Design review of the part built by this model. Coordinates are the model's own, in mm. A direction names the side the tool comes from. Coordinates: 2 decimals unless noted, no trailing zeros. Write each loop counter-clockwise with the first axis right and the second up, starting at its lowest first coordinate (ties: lowest second). Pieces come first, ordered by that corner, then holes. Notation, with made-up numbers: (11, 84.25) - (17, 84.25) arc R24 ccw to (17, 114.25) - close; hole circle Ø2 at (43.5, 42). An arc over 180 degrees is marked (long way). Use a Markdown table: item, result.
from build123d import *

# Parameters (mm, degrees)
BASE_FLANGE_DEPTH        = 7.5
NOTCH_CUT_DEPTH          = 26.568339797
EDGE_FLANGE1_DEPTH       = 7
M4_CLEARANCE_SLOT1_DEPTH = 1
HOLE1_OUTLINE_R          = 2.25
HOLE1_DEPTH              = 1


# Read off the part's stored shape, not the designer's step: M4 Clearance Slot1, Hole1
# Sheet-metal steps are written as plain solids
with BuildPart() as part:
    # Profile Sketch → Base Flange (new, symmetric)
    with BuildSketch(Plane(origin=(171.772586935, 0, 3.13889728), x_dir=(-1, 0, 0), z_dir=(0, 1, 0))):
        with BuildLine():
            Line((155.772586935, -3.13889728), (170.035986935, -3.13889728))
            ThreePointArc((170.035986935, -3.13889728), (171.263948571, -2.630258916), (171.772586935, -1.40229728))
            Line((171.772586935, -1.40229728), (171.772586935, 16.16110272))
            Line((171.772586935, 16.16110272), (170.772586935, 16.16110272))
            Line((170.772586935, 16.16110272), (170.772586935, -1.40229728))
            ThreePointArc((170.772586935, -1.40229728), (170.55684179, -1.923152135), (170.035986935, -2.13889728))
            Line((170.035986935, -2.13889728), (155.772586935, -2.13889728))
            Line((155.772586935, -2.13889728), (155.772586935, -3.13889728))
        make_face()
    extrude(amount=BASE_FLANGE_DEPTH, both=True)

    # Sketch1 → Notch Cut (cut, symmetric)
    with BuildSketch(Plane(origin=(1, 0, 0), x_dir=(0, 0, -1), z_dir=(1, 0, 0))):
        with BuildLine():
            Line((-10.3, -56.296391585), (-10.3, -7.5))
            ThreePointArc((-10.3, -7.5), (-11.3, -6.5), (-12.3, -7.5))
            Line((-12.3, -7.5), (-12.3, -56.296391585))
            Line((-12.3, -56.296391585), (-12.3, -153.889174754))
            Line((-12.3, -153.889174754), (-10.3, -153.889174754))
            Line((-10.3, -153.889174754), (-10.3, -56.296391585))
        make_face()
    notch_cut = extrude(amount=NOTCH_CUT_DEPTH, both=True, mode=Mode.SUBTRACT)

    # Edge-Flange1 section (across the edge) → Edge-Flange1 (add)
    with BuildSketch(Plane(origin=(0, -7.75, 12.3), x_dir=(0, 1, 0), z_dir=(0, 0, 1))):
        with BuildLine():
            Line((-1, 0.25), (-1, 1.75))
            Line((-1, 1.75), (0, 1.75))
            Line((0, 1.75), (0, 0.25))
            ThreePointArc((0, 0.25), (0.073223305, 0.073223305), (0.25, 0))
            Line((0.25, 0), (0.25, -1))
            ThreePointArc((0.25, -1), (-0.633883476, -0.633883476), (-1, 0.25))
        make_face()
    edge_flange1 = extrude(amount=EDGE_FLANGE1_DEPTH)

    # Alignment Tab Mirror: Notch Cut, Edge-Flange1 across plane
    add(notch_cut.mirror(Plane.ZX), mode=Mode.SUBTRACT)
    add(edge_flange1.mirror(Plane.ZX))

    # M4 Clearance Slot1 outline → M4 Clearance Slot1 (cut)
    with BuildSketch(Plane.XY):
        with BuildLine():
            Line((11.15, -1.1), (11.15, 1.1))
            ThreePointArc((11.15, 1.1), (9, 3.25), (6.85, 1.1))
            Line((6.85, 1.1), (6.85, -1.1))
            ThreePointArc((6.85, -1.1), (9, -3.25), (11.15, -1.1))
        make_face()
    extrude(amount=M4_CLEARANCE_SLOT1_DEPTH, mode=Mode.SUBTRACT)

    # Hole1 outline → Hole1 (cut)
    with BuildSketch(Plane.YZ):
        with Locations((0, 11.5)):
            Circle(HOLE1_OUTLINE_R)
    extrude(amount=HOLE1_DEPTH, mode=Mode.SUBTRACT)


solid = part.part
(1) Machinability: for faces 1 (the cylindrical face through (9.05, 3.25, 0.49)), 2 (the flat face through (16, 0.1, 0.5)), 3 (the flat face through (5.7, 7.5, 0.6)), 4 (the flat face through (0, -8, 12.3)), 5 (the flat face through (0, 0, 8)), which of the approach directions +Z, -Z, +X, -X, +Y, -Y give a long, thin tool a straight path to every point of the face, cutting with its end or side? Answer none if there is none.
Determined:
| item | result |
|---|---|
| face 1 | +Z, -Z |
| face 2 | +Z, -Z, +X, +Y, -Y |
| face 3 | -Z, +X, -X, +Y |
| face 4 | -Z, +X, -X, -Y |
| face 5 | +Z, -Z, -X |
(2) For L1, parallel to X at y = -5.5, z = 17.75; L2, parallel to Y at x = 0.75, z = 2.5, list the stretches that pass through material, from the lowest coordinate up. Write a range as from..to.
Determined:
| item | result |
|---|---|
| L1 | 0..1 |
| L2 | -7.5..7.5 |
(3) Take a section at D-D on y = -2.75. Write out the cut boundary in (x, z), and give its area (3 significant figures).
Determined:
| item | result |
|---|---|
| outline | (0, 1.74) arc R1.74 ccw to (1.74, 0) - (7.62, 0) - (7.62, 1) - (1.74, 1) arc R0.74 cw to (1, 1.74) - (1, 19.3) - (0, 19.3) - close; (10.38, 0) - (16, 0) - (16, 1) - (10.38, 1) - close |
| area | 31.0 mm2 |
(4) Draft analysis for pull direction Z (two halves, no side actions). For faces 6 (the flat face through (-1, -8.75, 16)), 7 (the cylindrical face through (0.52, 0.11, 0.5)), 8 (the cylindrical face through (0.49, -0.29, 13.73)), state which applies: +Z half, -Z half, draft (parallel to the pull), parting line (faces both ways), or undercut.
Determined:
| item | result |
|---|---|
| face 6 | draft |
| face 7 | -Z half |
| face 8 | undercut |
(5) Take a section at B-B on x = 9. Write out the cut boundary in (y, z), and give its area (3 significant figures).
Determined:
| item | result |
|---|---|
| outline | (-7.5, 0) - (-3.25, 0) - (-3.25, 1) - (-7.5, 1) - close; (3.25, 0) - (7.5, 0) - (7.5, 1) - (3.25, 1) - close |
| area | 8.50 mm2 |
(6) For pin 1 (0.6 mm diameter, centred on x = 0, y = -8.5, fed in from -Z); pin 2 (8 mm diameter, centred on x = 10.5, z = 8.5, fed in from +Y); pin 3 (7.5 mm diameter, centred on y = -2.5, z = 10, fed in from -X); pin 4 (7.5 mm diameter, centred on y = -2, z = 12, fed in from +X), all flat-tipped, find the tip position at first contact; note any pin that passes through.
Determined:
| item | result |
|---|---|
| pin 1 | z = 12.3 |
| pin 2 | through |
| pin 3 | x = 0 |
| pin 4 | x = 1 |
(7) Take a section at A-A on y = 0. Write out the cut boundary in (x, z).
Determined:
| item | result |
|---|---|
| outline | (0, 1.74) arc R1.74 ccw to (1.74, 0) - (6.85, 0) - (6.85, 1) - (1.74, 1) arc R0.74 cw to (1, 1.74) - (1, 9.25) - (0, 9.25) - close; (0, 13.75) - (1, 13.75) - (1, 19.3) - (0, 19.3) - close; (11.15, 0) - (16, 0) - (16, 1) - (11.15, 1) - close |
(8) Take a section at C-C on y = 5. Write out the cut boundary in (x, z).
Determined:
| item | result |
|---|---|
| outline | (0, 1.74) arc R1.74 ccw to (1.74, 0) - (16, 0) - (16, 1) - (1.74, 1) arc R0.74 cw to (1, 1.74) - (1, 19.3) - (0, 19.3) - close |
